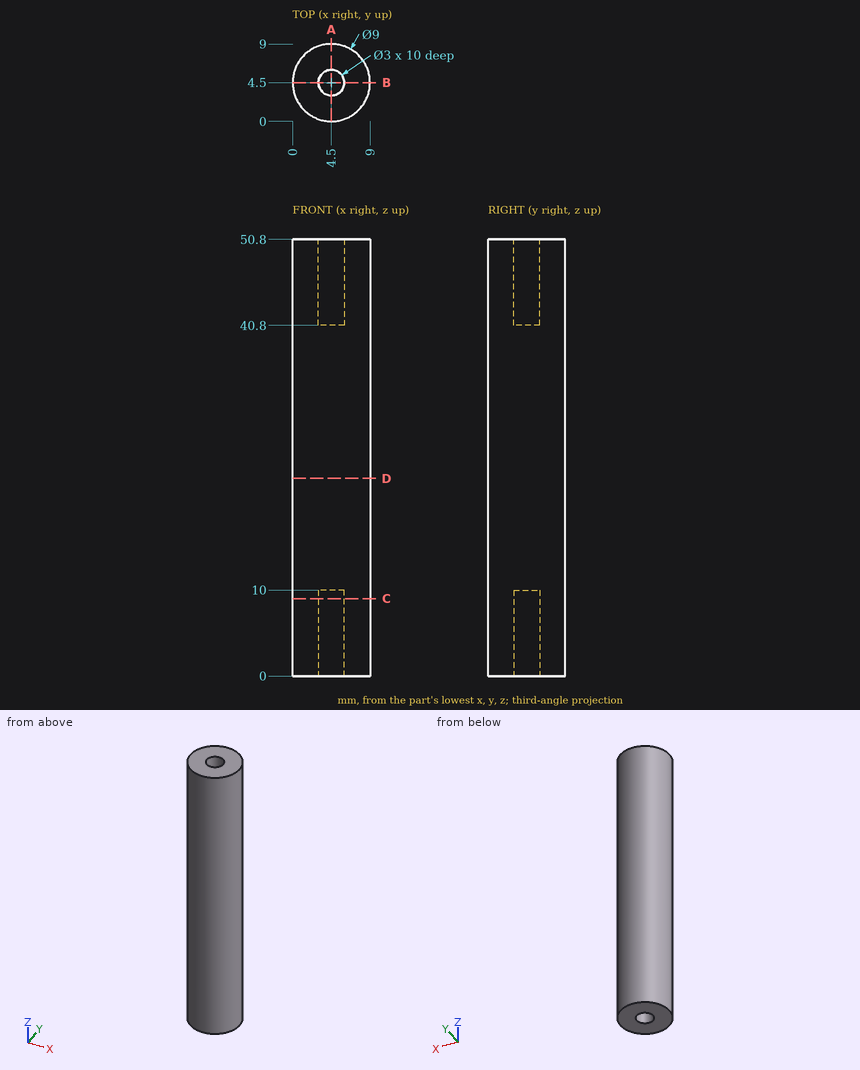
Drawing for the job (mm, zero at the part's lowest x, y, z). Round coordinates to 2 decimals unless told otherwise and drop trailing zeros. Loops run counter-clockwise (first coordinate to the right, second up) from the corner with the lowest first, then second, coordinate; pieces in that order, holes last. Notation, with made-up numbers: M 79.5,15 L 111.5,15 A26 cw 111.5,47 Z; hole C 79.5,85 d4. An arc over 180 degrees is marked long. Use a Markdown table: item, result. Add a question column.
(1) Drill centre lines: line 1 (Y direction, x = 4.5, z = 41); line 2 (Z direction, x = 5.5, y = 5.5); line 3 (Y direction, x = 5, z = 2). Where is each one in solid material? Low to high.
(2) Cut at A-A (x = 4.5). Give the cut face in (y, z), and give its area (3 significant figures).
(3) Cut at C-C (z = 9). Give the cut face in (x, y).
(4) Cut at D-D (z = 23). Give the cut face in (x, y).
(5) Flat gauge pins, fed straight in: pin 1 (1 mm diameter, centred on y = 6.5, z = 43, fed in from +X); pin 2 (1 mm diameter, centred on x = 4.5, y = 4.5, fed in from -Z); pin 3 (1.5 mm diameter, centred on y = 8, z = 36.5, fed in from +X). Where does each tip first touch, or does it go through?
Geometry says:
| question | item | result |
|---|---|---|
| 1 | line 1 | y = 0 to 3, 6 to 9 |
| 1 | line 2 | z = 10 to 40.8 |
| 1 | line 3 | y = 0.03 to 3.09, 5.91 to 8.97 |
| 2 | outline | M 0,0 L 3,0 L 3,10 L 6,10 L 6,0 L 9,0 L 9,50.8 L 6,50.8 L 6,40.8 L 3,40.8 L 3,50.8 L 0,50.8 Z |
| 2 | area | 397 mm² |
| 3 | outline | C 4.5,4.5 d9; hole C 4.5,4.5 d3 |
| 4 | outline | C 4.5,4.5 d9 |
| 5 | pin 1 | stops at x = 8.74 |
| 5 | pin 2 | stops at z = 10 |
| 5 | pin 3 | stops at x = 8.06 |
